Job drawing, mm, ordinate dimensions from the low corner. One solid piece. A direction names the side the tool comes from. Round coordinates to 2 decimals unless told otherwise and drop trailing zeros. Loops run counter-clockwise (first coordinate to the right, second up) from the corner with the lowest first, then second, coordinate; pieces in that order, holes last.
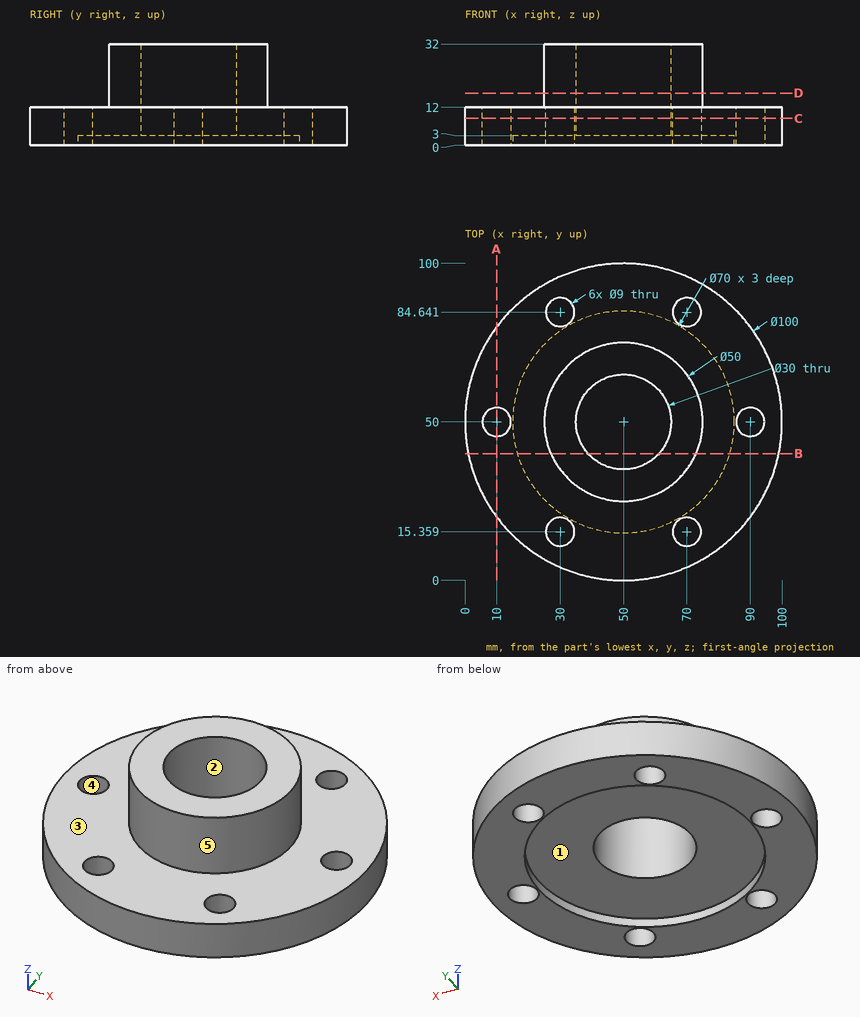
Item 1: Probe line 1 (Y direction, x = 49.5, z = 3.5); line 2 (Y direction, x = 30, z = 9); line 3 (Y direction, x = 71, z = 10). List the from-to ranges inside material, lowest first.
Answers follow:
line 1: y = 0 to 35.01, 64.99 to 100
line 2: y = 4.17 to 10.86, 19.86 to 80.14, 89.14 to 95.83
line 3: y = 4.62 to 10.97, 19.75 to 80.25, 89.03 to 95.38
Item 2: Two-plate mould, pull along X, no slides. Class the marked faces 3, 4 and 5: released by +X, released by -X, zero draft, split by the parting line, or undercut.
Answers follow:
face 3: zero draft
face 4: undercut
face 5: split by the parting line
Item 3: 3-axis set-ups, long thin cutter, end or side, ignore diameter. For the marked faces 1 and 2: which of +Z, -Z, +X, -X, +Y, -Y reach the whole face in a straight line?
Answers follow:
face 1: -Z
face 2: +Z, -Z
Item 4: Cut at B-B, the plane y = 40. Give the cut face in (x, z), plus the area to 3 significant figures.
Answers follow:
outline: (1.01, 0) - (16.46, 0) - (16.46, 3) - (38.82, 3) - (38.82, 32) - (27.09, 32) - (27.09, 12) - (1.01, 12) - close; (61.18, 3) - (83.54, 3) - (83.54, 0) - (98.99, 0) - (98.99, 12) - (72.91, 12) - (72.91, 32) - (61.18, 32) - close
area: 1,240 mm2
Item 5: Flat gauge pins, fed straight in: P1, Ø12, axis at x = 77, z = 27, coming from the +Y side; P2, Ø10, axis at y = 45, z = 22, coming from the -X side; P3, Ø11.5, axis at x = 30, y = 84.64, coming from the +Z side. Where does each tip first touch, or does it go through?
Answers follow:
P1: stops at y = 63.56
P2: stops at x = 25
P3: stops at z = 12
Item 6: Cut at A-A, the plane x = 10. Give the cut face in (y, z), plus the area to 3 significant figures.
Answers follow:
outline: (20, 0) - (45.5, 0) - (45.5, 12) - (20, 12) - close; (54.5, 0) - (80, 0) - (80, 12) - (54.5, 12) - close
area: 612 mm2
Item 7: Cut at D-D, the plane z = 16.5. Give the cut face in (x, y).
Answers follow:
outline: circle Ø50 at (50, 50); hole circle Ø30 at (50, 50)
Item 8: Cut at C-C, the plane z = 8.5. Give the cut face in (x, y), plus the area to 3 significant figures.
Answers follow:
outline: circle Ø100 at (50, 50); hole circle Ø9 at (10, 50); hole circle Ø9 at (30, 15.36); hole circle Ø9 at (30, 84.64); hole circle Ø30 at (50, 50); hole circle Ø9 at (70, 15.36); hole circle Ø9 at (70, 84.64); hole circle Ø9 at (90, 50)
area: 6,770 mm2
